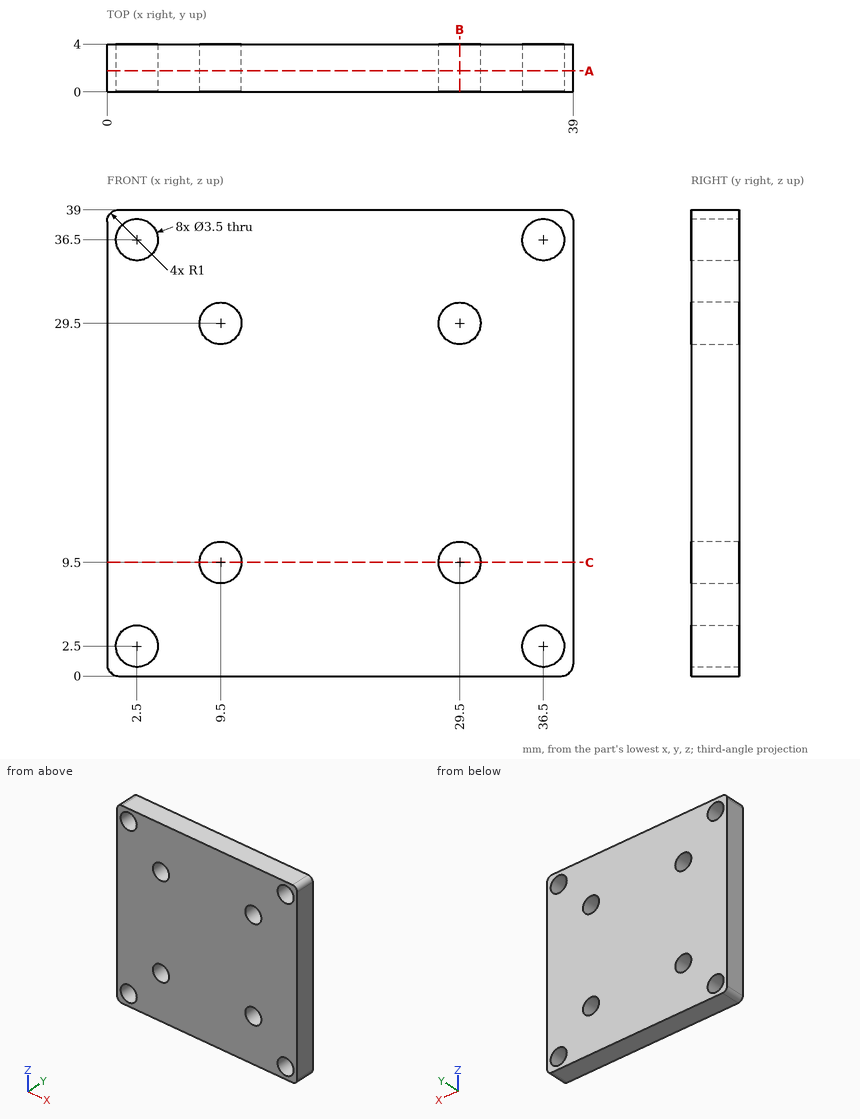
Study the drawing (mm; zero at the part's minimum x, y, z) and answer. Give positions to 0.01 mm unless a question says otherwise; leave off trailing zeros. Order: outer loops, then holes, each group sorted by start corner. A loop starts at its lowest first (then second) coordinate and runs counter-clockwise, first axis right, second up. Notation, with made-up numbers: (60, -30) - (89, -30) arc R22 cw to (89, -18) - close; hole circle Ø8 at (-10, 21). An arc over 180 degrees is marked (long way). Answer in a Markdown table with one row per item. Add a question column.
Q1. The part is cut by section C-C (z = 9.5). Determine the outline of the cut face in (x, y).
Q2. The part is cut by section B-B (x = 29.5). Determine the outline of the cut face in (y, z), then the cut area to 3 significant figures.
Q3. Find the intervals of material crossed by line 1 along X through (y, z) = (3.05, 29.5); line 2 along Z through (x, y) = (37, 3.4); line 3 along Z through (x, y) = (35.5, 0.95), in increasing order. Write a range as [from, to].
Q4. Given P1, Ø3, axis at x = 36.5, z = 2.5, coming from the +Y side, flat-ended and moving along its own axis, determine where the tip first touches the part or whether it passes through.
Q5. The part is cut by section A-A (y = 1.75). Give the number of separate pieces and of enclosed holes in the cut face, then the cut area to 3 significant figures.
Determined:
| question | item | result |
|---|---|---|
| 1 | outline | (0, 0) - (7.75, 0) - (7.75, 4) - (0, 4) - close; (11.25, 0) - (27.75, 0) - (27.75, 4) - (11.25, 4) - close; (31.25, 0) - (39, 0) - (39, 4) - (31.25, 4) - close |
| 2 | outline | (0, 0) - (4, 0) - (4, 7.75) - (0, 7.75) - close; (0, 11.25) - (4, 11.25) - (4, 27.75) - (0, 27.75) - close; (0, 31.25) - (4, 31.25) - (4, 39) - (0, 39) - close |
| 2 | area | 128 mm² |
| 3 | line 1 | x = [0, 7.75], [11.25, 27.75], [31.25, 39] |
| 3 | line 2 | z = [0, 0.82], [4.18, 34.82], [38.18, 39] |
| 3 | line 3 | z = [0, 1.06], [3.94, 35.06], [37.94, 39] |
| 4 | P1 | passes through |
| 5 | separate pieces | 1 |
| 5 | enclosed holes | 8 |
| 5 | area | 1,440 mm² |
